Design review of the part built by this model. Coordinates are the model's own, in mm. Face numbers are marked on the shaded views. A direction names the side the tool comes from. Round coordinates to 2 decimals unless told otherwise and drop trailing zeros. Loops run counter-clockwise (first coordinate to the right, second up) from the corner with the lowest first, then second, coordinate; pieces in that order, holes last. Notation, with made-up numbers: (-18, 18.25) - (-9, 18.25) arc R22 cw to (-9, 53.25) - close; hole circle Ø9 at (-15.75, 11.25). An arc over 180 degrees is marked (long way). Use one line per item in the form item = value. Start each with the question number.
(1) We need section B-B, the plane z = 4.5. Write out the cut boundary in (x, y), then the cut area to 3 significant figures.
(2) Wall thickness on probe 1 along Y at (x, z) = (-11.25, 11.25); probe 2 along Y at (x, z) = (-11.25, 1.5); probe 3 along X at (y, z) = (-15, 18.75): over which ranges is each line inside the solid? List them lowest first. Write a range as [from, to].
(3) We need section D-D, the plane y = -11.25. Write out the cut boundary in (x, z).
(4) The part is to be moulded in two halves that separate along Y. For the marked faces 1, 2, 3 and 4, say which applies: released by +Y, released by -Y, zero draft, split by the parting line, or undercut.
(5) For pin 1 (6.5 mm diameter, centred on x = -11.25, y = -14.75, fed in from +Z), flat-tipped, find the tip position at first contact; note if it passes through.
(6) Machinability: for the marked faces 5 and 6, which of the approach directions +Z, -Z, +X, -X, +Y, -Y give a long, thin tool a straight path to every point of the face, cutting with its end or side? Answer none if there is none.
(7) We need section C-C, the plane x = -9. Write out the cut boundary in (y, z), then the cut area to 3 significant figures.
(8) We need section A-A, the plane y = -14.75. Write out the cut boundary in (x, z).
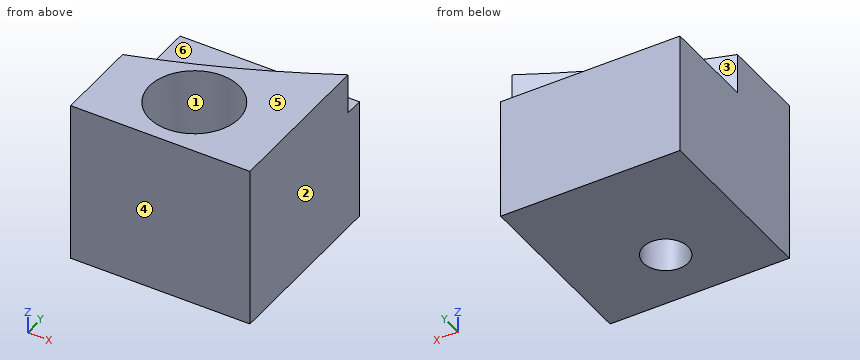
from build123d import *

# Parameters (mm, degrees)
F0_W     = 22
F0_H     = 22
F0_R     = 2.75
F1_DEPTH = 20
F2_R     = 5.5
F2_R_2   = 2.75
F3_DEPTH = 15
F5_DEPTH = 5


with BuildPart() as f1:
    # F0 (on Top) → F1 (new body)
    with BuildSketch(Plane.XY):
        with Locations((-11, -11)):
            Rectangle(F0_W, F0_H)
        with Locations((-11.25, -14.75)):
            Circle(F0_R, mode=Mode.SUBTRACT)
    extrude(amount=F1_DEPTH)

    # F2 (on face) → F3 (cut)
    with BuildSketch(Plane.XY.offset(20)):
        with Locations((-11.25, -14.75)):
            Circle(F2_R)
        with Locations((-11.25, -14.75)):
            Circle(F2_R_2, mode=Mode.SUBTRACT)
    extrude(amount=-F3_DEPTH, mode=Mode.SUBTRACT)

    # F4 (on face) → F5 (cut)
    with BuildSketch(Plane.XY.offset(20)):
        with BuildLine():
            Line((0, 0), (-22, 0))
            Line((-22, 0), (-22, -11.5693575736))
            ThreePointArc((-22, -11.5693575736), (-10.7684476262, -7.4750665799), (0, -2.2835809364))
            Line((0, -2.2835809364), (0, 0))
        make_face()
    extrude(amount=-F5_DEPTH, mode=Mode.SUBTRACT)


solid = f1.part
Data:
q1.outline = (-22, -22) - (0, -22) - (0, 0) - (-22, 0) - close; hole circle Ø5.5 at (-11.25, -14.75)
q1.area = 460 mm^2
q2.probe_1 = [-22, -20.25], [-9.25, 0]
q2.probe_2 = [-22, -17.5], [-12, 0]
q2.probe_3 = [-22, -16.74], [-5.76, 0]
q3.outline = (-22, 0) - (0, 0) - (0, 20) - (-7.01, 20) - (-7.01, 5) - (-15.49, 5) - (-15.49, 20) - (-20.98, 20) - (-20.98, 15) - (-22, 15) - close
q4.face_1 = undercut
q4.face_2 = zero draft
q4.face_3 = released by +Y
q4.face_4 = released by -Y
q5.pin_1 = 5
q6.face_5 = +Z, +X, -X, +Y, -Y
q6.face_6 = +Z, -X, +Y
q7.outline = (-22, 0) - (-16.33, 0) - (-16.33, 5) - (-19.77, 5) - (-19.77, 20) - (-22, 20) - close; (-13.17, 0) - (0, 0) - (0, 15) - (-6.71, 15) - (-6.71, 20) - (-9.73, 20) - (-9.73, 5) - (-13.17, 5) - close
q7.area = 240 mm^2
q8.outline = (-22, 0) - (-14, 0) - (-14, 5) - (-16.75, 5) - (-16.75, 20) - (-22, 20) - close; (-8.5, 0) - (0, 0) - (0, 20) - (-5.75, 20) - (-5.75, 5) - (-8.5, 5) - close
